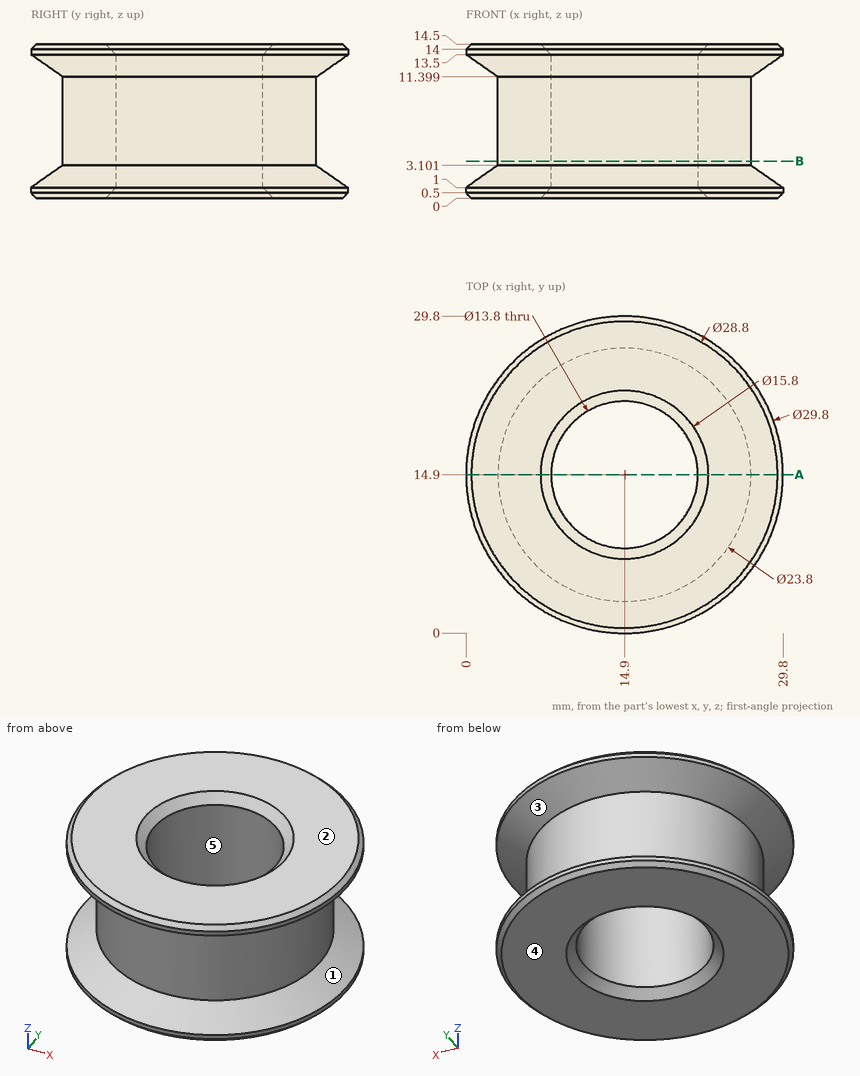
Geometry: see drawing. Coordinates: mm, zero at the bounding-box minimum. A direction names the side the tool comes from. Round coordinates to 2 decimals unless told otherwise and drop trailing zeros. Loops run counter-clockwise (first coordinate to the right, second up) from the corner with the lowest first, then second, coordinate; pieces in that order, holes last. Notation, with made-up numbers: (48, 83) - (63, 83) arc R19 ccw to (63, 119) - close; hole circle Ø8 at (71, 54.5). An arc over 180 degrees is marked (long way). One line per item, written item: value. Start each with the question number.
(1) Section A-A, the plane y = 14.9. Return loops of the section in (x, z).
(2) Access query for the marked faces 1 and 2. Directions: +Z, -Z, +X, -X, +Y, -Y. A direction counts if a zero-diameter tool reaches every point of the face in a straight line with its end or side. Return the directions, or none.
(3) Ray query, line 1 (Y direction, x = 14.9, z = 5.75); line 2 (Y direction, x = 20.25, z = 10.75) (1 decimal); line 3 (X direction, y = 11.5, z = 8.25) (1 decimal). Return the intervals inside material, ascending. Write a range as [from, to].
(4) Section B-B, the plane z = 3.5. Return loops of the section in (x, y).
(5) Contact query for flat-ended pins moving along their axis: P1, Ø12.5, axis at x = 14.9, y = 14.9, coming from the -Z side; P2, Ø8, axis at y = 22, z = 2, coming from the +X side; P3, Ø3, axis at x = 10, z = 10.5, coming from the -Y side (1 decimal). Output: stop coordinate, or through.
(6) Draft query along X for the marked faces 3, 4 and 5. Return one class per face: +X half, -X half, draft (parallel to the pull), parting line (faces both ways), or undercut.
Results below:
1. outline: (0, 0.5) - (0.5, 0) - (7, 0) - (8, 1) - (8, 13.5) - (7, 14.5) - (0.5, 14.5) - (0, 14) - (0, 13.5) - (3, 11.4) - (3, 3.1) - (0, 1) - close; (21.8, 1) - (22.8, 0) - (29.3, 0) - (29.8, 0.5) - (29.8, 1) - (26.8, 3.1) - (26.8, 11.4) - (29.8, 13.5) - (29.8, 14) - (29.3, 14.5) - (22.8, 14.5) - (21.8, 13.5) - close
2. face 1: none
2. face 2: +Z, +X, -X, +Y, -Y
3. line 1: [3, 8], [21.8, 26.8]
3. line 2: [4.3, 10.5], [19.3, 25.5]
3. line 3: [3.5, 8.9], [20.9, 26.3]
4. outline: circle Ø23.8 at (14.9, 14.9); hole circle Ø13.8 at (14.9, 14.9)
5. P1: through
5. P2: x = 29.45
5. P3: y = 3
6. face 3: parting line
6. face 4: draft
6. face 5: undercut
